For this review, take the finished solid that the model builds, in its own axes (mm). A direction names the side the tool comes from. Round coordinates to 2 decimals unless told otherwise and drop trailing zeros. Write each loop counter-clockwise with the first axis right and the second up, starting at its lowest first coordinate (ties: lowest second). Pieces come first, ordered by that corner, then holes.
from build123d import *

# Parameters (mm, degrees)
F1_DEPTH       = 82.55
F4_D           = 8.73125
F4_DEPTH       = 25.4
F4_TIP         = 2.6231321399
F4_ON_F3_D     = 8.73125
F4_ON_F3_DEPTH = 25.4
F4_ON_F3_TIP   = 2.6231321399
F5_R           = 5.08


with BuildPart() as f1:
    # F0 (on Front) → F1 (new body)
    with BuildSketch(Plane.XZ):
        Polygon((-38.1, 0), (0, 0), (0, 153.3652), (-18.0848, 153.3652), (-38.1, 133.35), align=None)
    extrude(amount=F1_DEPTH)

    # F4
    with Locations(Plane(origin=(-85.725, 0, 85.725), x_dir=(0, -1, 0), z_dir=(-0.7071067812, 0, 0.7071067812))):
        with Locations((73.025, 81.5048045548), (9.525, 81.5048045548)):
            Hole(F4_D / 2, depth=F4_DEPTH)
            with Locations((0, 0, -(F4_DEPTH + F4_TIP / 2))):  # 118° drill point
                Cone(0, F4_D / 2, F4_TIP, mode=Mode.SUBTRACT)

    # F4 on F3
    with Locations(Plane(origin=(0, 0, 0), x_dir=(1, 0, 0), z_dir=(0, 0, -1))):
        with Locations((-19.05, 73.025), (-19.05, 9.525)):
            Hole(F4_ON_F3_D / 2, depth=F4_ON_F3_DEPTH)
            with Locations((0, 0, -(F4_ON_F3_DEPTH + F4_ON_F3_TIP / 2))):  # 118° drill point
                Cone(0, F4_ON_F3_D / 2, F4_ON_F3_TIP, mode=Mode.SUBTRACT)

    # F5
    f5_edges = [f1.edges().sort_by_distance(p)[0] for p in [
        (-38.1, -41.275, 133.35),
        (-18.0848, -41.275, 153.3652),
        (0, -41.275, 153.3652),
    ]]
    fillet(f5_edges, radius=F5_R)


solid = f1.part
(1) Mouldability with a two-part tool opening along Z and no side actions: class faces 1 (the face through (-8.237, -72.466, 124.227)), 2 (the face through (-20.86, -76.49, 132.37)), 3 (the face through (-27.97, -40.7, 143.48)), 4 (the face through (0, -41, 73)) as pulls with the +Z half, pulls with the -Z half, needs draft (parallel to the pull), parting line crosses it, or undercut.
Geometry check:
face 1: undercut
face 2: undercut
face 3: pulls with the +Z half
face 4: needs draft
(2) For faces 5 (the face through (-23.1, -71.4, 12.9)), 6 (the face through (-8.068, -9.426, 124.396)), 7 (the face through (-37.724, -41.853, 133.164)), list the 3-axis set-ups (+Z, -Z, +X, -X, +Y, -Y) from which the entire face can be reached by the end or side of a thin tool; tool diameter is ignored.
Geometry check:
face 5: -Z
face 6: none
face 7: +Z, -X, +Y, -Y
(3) For pin 1 Ø10 at (x, y) = (-33.5, -61) entering from +Z; pin 2 Ø4 at (x, y) = (-28, -29.5) entering from +Z, all flat-tipped, find the tip position at first contact; note any pin that passes through.
Geometry check:
pin 1: stops at z = 142.95
pin 2: stops at z = 145.45
(4) For line 1 along Y through (x, z) = (-19.05, 7.25); line 2 along Y through (x, z) = (-16.5, 126); line 3 along Z through (x, y) = (-1.5, -39), list the stretches that pass through material, from the lowest coordinate up.
Geometry check:
line 1: y = -82.55 to -77.39, -68.66 to -13.89, -5.16 to 0
line 2: y = -82.55 to -74.59, -71.46 to -11.09, -7.96 to 0
line 3: z = 0 to 151.89
(5) We need section A-A, the plane y = -53.5. Give the boundary of the cut face in (x, z), and give its area (3 significant figures).
Geometry check:
outline: (-38.1, 0) - (0, 0) - (0, 148.29) arc R5.08 ccw to (-5.08, 153.37) - (-15.98, 153.37) arc R5.08 ccw to (-19.57, 151.88) - (-36.61, 134.84) arc R5.08 ccw to (-38.1, 131.25) - close
area: 5,640 mm2
(6) We need section B-B, the plane z = 16. Give the boundary of the cut face in (x, y) (3 decimals).
Geometry check:
outline: (-38.1, -82.55) - (0, -82.55) - (0, 0) - (-38.1, 0) - close; hole circle Ø8.731 at (-19.05, -73.025); hole circle Ø8.731 at (-19.05, -9.525)
